from build123d import *

# Parameters (mm, degrees)
F0_W     = 215.9
F0_H     = 139.7
F0_R     = 3.175
F1_DEPTH = 6.35


with BuildPart() as f1:
    # F0 (on Right) → F1 (new body)
    with BuildSketch(Plane.YZ):
        with Locations((107.95, 69.85)):
            Rectangle(F0_W, F0_H)
        with Locations((12.7, 127)):
            Circle(F0_R, mode=Mode.SUBTRACT)
        with BuildLine():
            Line((204.443743, 120.772994), (13.689743, 82.672994))
            ThreePointArc((13.689743, 82.672994), (6.218994, 87.656257), (11.202257, 95.127006))
            Line((11.202257, 95.127006), (201.956257, 133.227006))
            ThreePointArc((201.956257, 133.227006), (209.427006, 128.243743), (204.443743, 120.772994))
        make_face(mode=Mode.SUBTRACT)
    extrude(amount=F1_DEPTH)


solid = f1.part
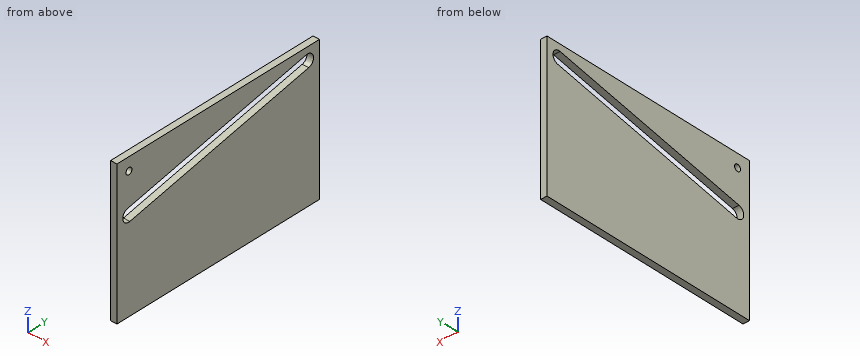
Design review of the part built by this model. Coordinates are the model's own, in mm. Coordinates: 2 decimals unless noted, no trailing zeros. Order: outer loops, then holes, each group sorted by start corner. A loop starts at its lowest first (then second) coordinate and runs counter-clockwise, first axis right, second up.
Item 1: For pin 1 Ø3 at (x, y) = (1.5, 144.5) entering from -Z, flat-tipped, find the tip position at first contact; note if it passes through.
Item 2: For line 1 (Z direction, x = 2.25, y = 12.7) (3 decimals); line 2 (Z direction, x = 1, y = 39); line 3 (Z direction, x = 0.5, y = 33), list the stretches that pass through material, from the lowest coordinate up.
Item 3: Take a section at D-D, the plane z = 127. Write out the cut boundary in (x, y) (3 decimals).
Item 4: Take a section at A-A, the plane x = 5.25. Write out the cut boundary in (y, z) (3 decimals).
Item 5: Take a section at B-B, the plane z = 88.9. Write out the cut boundary in (x, y), then the cut area to 3 significant figures.
Item 6: Take a section at C-C, the plane y = 21. Write out the cut boundary in (x, z).
The answers:
1. pin 1: stops at z = 0
2. line 1: z = 0 to 82.555, 95.426 to 123.825, 130.175 to 139.7
2. line 2: z = 0 to 87.73, 100.68 to 139.7
2. line 3: z = 0 to 86.53, 99.48 to 139.7
3. outline: (0, 0) - (6.35, 0) - (6.35, 9.525) - (0, 9.525) - close; (0, 15.875) - (6.35, 15.875) - (6.35, 170.78) - (0, 170.78) - close; (0, 209.55) - (6.35, 209.55) - (6.35, 215.9) - (0, 215.9) - close
4. outline: (0, 0) - (215.9, 0) - (215.9, 139.7) - (0, 139.7) - close; hole circle Ø6.35 at (12.7, 127); hole (11.202, 95.127) arc R6.35 ccw to (13.69, 82.673) - (204.444, 120.773) arc R6.35 ccw to (201.956, 133.227) - close
5. outline: (0, 0) - (6.35, 0) - (6.35, 6.1) - (0, 6.1) - close; (0, 44.87) - (6.35, 44.87) - (6.35, 215.9) - (0, 215.9) - close
5. area: 1,120 mm2
6. outline: (0, 0) - (6.35, 0) - (6.35, 84.13) - (0, 84.13) - close; (0, 97.08) - (6.35, 97.08) - (6.35, 139.7) - (0, 139.7) - close
